from build123d import *

# Parameters (mm, degrees)
F1_DEPTH = 20
F3_D     = 10
F4_R     = 18
F5_DEPTH = 30
F7_D     = 14
F7_DEPTH = 18
F7_TIP   = 4.2060243332


with BuildPart() as f1:
    # F0 (on Top) → F1 (new body)
    with BuildSketch(Plane.XY):
        with BuildLine():
            ThreePointArc((39.2857142857, -9.0350790291), (29.6547751618, -8.4515425473), (25, 0))
            ThreePointArc((25, 0), (21.1288563682, -13.3630620956), (10.7142857143, -22.5876975726))
            Line((10.7142857143, -22.5876975726), (39.2857142857, -9.0350790291))
        make_face()
        with BuildLine():
            ThreePointArc((10.7142857143, 22.5876975726), (21.1288563682, 13.3630620956), (25, 0))
            ThreePointArc((25, 0), (29.6547751618, 8.4515425473), (39.2857142857, 9.0350790291))
            Line((39.2857142857, 9.0350790291), (10.7142857143, 22.5876975726))
        make_face()
        with BuildLine():
            ThreePointArc((-25, 0), (-21.1288563682, 13.3630620956), (-10.7142857143, 22.5876975726))
            Line((-10.7142857143, 22.5876975726), (-39.2857142857, 9.0350790291))
            ThreePointArc((-39.2857142857, 9.0350790291), (-29.6547751618, 8.4515425473), (-25, 0))
        make_face()
        with BuildLine():
            Line((-39.2857142857, -9.0350790291), (-10.7142857143, -22.5876975726))
            ThreePointArc((-10.7142857143, -22.5876975726), (-21.1288563682, -13.3630620956), (-25, 0))
            ThreePointArc((-25, 0), (-29.6547751618, -8.4515425473), (-39.2857142857, -9.0350790291))
        make_face()
        with BuildLine():
            ThreePointArc((-39.2857142857, -9.0350790291), (-29.6547751618, -8.4515425473), (-25, 0))
            ThreePointArc((-25, 0), (-29.6547751618, 8.4515425473), (-39.2857142857, 9.0350790291))
            ThreePointArc((-39.2857142857, 9.0350790291), (-45, 0), (-39.2857142857, -9.0350790291))
        make_face()
        with BuildLine():
            ThreePointArc((39.2857142857, 9.0350790291), (29.6547751618, 8.4515425473), (25, 0))
            ThreePointArc((25, 0), (29.6547751618, -8.4515425473), (39.2857142857, -9.0350790291))
            ThreePointArc((39.2857142857, -9.0350790291), (43.4515425473, -5.3452248382), (45, 0))
            ThreePointArc((45, 0), (43.4515425473, 5.3452248382), (39.2857142857, 9.0350790291))
        make_face()
        with BuildLine():
            ThreePointArc((10.7142857143, -22.5876975726), (21.1288563682, -13.3630620956), (25, 0))
            ThreePointArc((25, 0), (21.1288563682, 13.3630620956), (10.7142857143, 22.5876975726))
            ThreePointArc((10.7142857143, 22.5876975726), (0, 25), (-10.7142857143, 22.5876975726))
            ThreePointArc((-10.7142857143, 22.5876975726), (-21.1288563682, 13.3630620956), (-25, 0))
            ThreePointArc((-25, 0), (-21.1288563682, -13.3630620956), (-10.7142857143, -22.5876975726))
            ThreePointArc((-10.7142857143, -22.5876975726), (0, -25), (10.7142857143, -22.5876975726))
        make_face()
    extrude(amount=F1_DEPTH)

    # F3 (through all)
    with Locations(Plane(origin=(0, 0, 0), x_dir=(1, 0, 0), z_dir=(0, 0, -1))):
        with Locations((-35, 0), (35, 0)):
            Hole(F3_D / 2)

    # F4 (on face) → F5 (join)
    with BuildSketch(Plane.XY.offset(20)):
        Circle(F4_R)
    extrude(amount=F5_DEPTH)

    # F7
    with Locations(Plane.XY.offset(50)):
        with Locations((0, 0)):
            Hole(F7_D / 2, depth=F7_DEPTH)
            with Locations((0, 0, -(F7_DEPTH + F7_TIP / 2))):  # 118° drill point
                Cone(0, F7_D / 2, F7_TIP, mode=Mode.SUBTRACT)


solid = f1.part
Check sheet for the modelled part. Datum: model origin and axes. Units: mm. A direction names the side the tool comes from. Round coordinates to 2 decimals unless told otherwise and drop trailing zeros. Write each loop counter-clockwise with the first axis right and the second up, starting at its lowest first coordinate (ties: lowest second). Pieces come first, ordered by that corner, then holes. Notation, with made-up numbers: (79, 78.5) -> (138, 78.5) arc R34 cw to (138, 114.5) -> close; hole circle Ø2 at (6.25, -30.75). An arc over 180 degrees is marked (long way). Answer as CSV lines item,"result". Start each with the question number.
1) Go/stop test with flat-tipped pins: P1, Ø2, axis at y = -6.5, z = 5, coming from the +X side; P2, Ø1.5, axis at x = -15.5, z = 14.5, coming from the -Y side; P3, Ø10, axis at x = -25, z = 24, coming from the +Y side. Record where each tip stops, or that it passes through.
2) Section check C-C on z = 36.5. Enter the section's corners in (x, y), and give its area (3 significant figures).
3) Section check D-D on y = 11. Enter the section's corners in (x, z).
4) Section check B-B on x = -35. Enter the section's corners in (y, z).
5) Tool access check on faces 5 (the cylindrical face through (-2.343, 17.847, 34.79)), 6 (the cylindrical face through (0, 25, 10)). Record the directions out of +Z, -Z, +X, -X, +Y, -Y that give a thin tool (end or side, any length) a straight path to the whole face; none if there is none.
6) Release check for a two-part mould opening along Y. For faces 1 (the cylindrical face through (-6.466, -2.681, 40.874)), 2 (the flat face through (-25.2, -15.717, 9.86)), 3 (the cylindrical face through (-45, 0, 10)), 4 (the conical face through (-0.264, -1.187, 28.524)) record: pulls with the +Y half, pulls with the -Y half, needs draft (parallel to the pull), parting line crosses it, or undercut.
7) Section check A-A on z = 12. Enter the section's corners in (x, y), and give its area (3 significant figures).
8) Material ranges on line 1 (Y direction, x = 0, z = 40.25); line 2 (Z direction, x = -26, y = 9.5); line 3 (Y direction, x = 35, z = 15), recorded low to high. Write a range as from..to.
Found:
1,P1,"stops at x = 43.35"
1,P2,"stops at y = -20.67"
1,P3,"stops at y = 17.23"
2,outline,"circle Ø36 at (0, 0); hole circle Ø14 at (0, 0)"
2,area,"864 mm^2"
3,outline,"(-35.14, 0) -> (35.14, 0) -> (35.14, 20) -> (14.25, 20) -> (14.25, 50) -> (-14.25, 50) -> (-14.25, 20) -> (-35.14, 20) -> close"
4,outline,"(-11.07, 0) -> (-5, 0) -> (-5, 20) -> (-11.07, 20) -> close; (5, 0) -> (11.07, 0) -> (11.07, 20) -> (5, 20) -> close"
5,face 5,"+Z"
5,face 6,"+Z, -Z, +Y"
6,face 1,"undercut"
6,face 2,"pulls with the -Y half"
6,face 3,"parting line crosses it"
6,face 4,"undercut"
7,outline,"(-39.29, -9.04) -> (-10.71, -22.59) arc R25 ccw to (10.71, -22.59) -> (39.29, -9.04) arc R10 ccw to (39.29, 9.04) -> (10.71, 22.59) arc R25 ccw to (-10.71, 22.59) -> (-39.29, 9.04) arc R10 ccw to start; hole circle Ø10 at (-35, 0); hole circle Ø10 at (35, 0)"
7,area,"2,840 mm^2"
8,line 1,"y = -18..-7, 7..18"
8,line 2,"z = 0..20"
8,line 3,"y = -11.07..-5, 5..11.07"
